Autodesk Inventor part; units mm, degrees
ref_plane "YZ Plane" through (0, 0, 0) normal (1, 0, 0) x (0, 1, 0)
ref_plane "XZ Plane" through (0, 0, 0) normal (0, 1, 0) x (-1, 0, 0)
ref_plane "XY Plane" through (0, 0, 0) normal (0, 0, 1) x (1, 0, 0)
sketch "Sketch1" plane through (0, 0, 0) normal (1, 0, 0) x (0, 1, 0)
  line L0 (-1143.0823, -35.5862) -> (966.1492, 732.1113)
  line L1 (-1143.0823, -35.5862) -> (-1143.0823, -135.5862)
  line L2 (966.1492, 732.1113) -> (966.1492, 632.1113)
  line L3 (-1143.0823, -135.5862) -> (966.1492, 632.1113)
  point P0 (0, 0)
  point P1 (1136.1492, -719.9922)
extrude "Extrusion1" add sketch "Sketch1" along normal blind 1696
sketch "Sketch2" plane through (1696, 0, 0) normal (1, 0, 0) x (0, 0, -1)
  line L0 (-632.1113, 966.1492) -> (-732.1113, 966.1492)
  line L1 (-732.1113, 966.1492) -> (-595.3032, 590.2722)
  line L2 (-595.3032, 590.2722) -> (-585.3032, 590.2722)
  line L3 (-585.3032, 590.2722) -> (-578.4628, 571.4783)
  line L4 (-578.4628, 571.4783) -> (-588.4628, 571.4783)
  line L5 (-588.4628, 571.4783) -> (-451.6548, 195.6013)
  line L6 (-732.1113, 966.1492) -> (35.5862, -1143.0823)
  line L7 (-451.6548, 195.6013) -> (-441.6548, 195.6013)
  line L8 (-441.6548, 195.6013) -> (-434.8144, 176.8074)
  line L9 (-434.8144, 176.8074) -> (-445.1891, 177.8369)
  line L10 (-445.1891, 177.8369) -> (-308.381, -198.0401)
  line L11 (-308.381, -198.0401) -> (-298.381, -198.0401)
  line L12 (-298.381, -198.0401) -> (-291.5406, -216.834)
  line L13 (-291.5406, -216.834) -> (-301.5406, -216.834)
  line L14 (-301.5406, -216.834) -> (-164.7326, -592.711)
  line L15 (-164.7326, -592.711) -> (-154.7326, -592.711)
  line L16 (-154.7326, -592.711) -> (-147.8921, -611.5049)
  line L17 (-147.8921, -611.5049) -> (-157.8921, -611.5049)
  line L18 (-157.8921, -611.5049) -> (-21.0841, -987.3819)
  line L19 (-21.0841, -987.3819) -> (-11.0841, -987.3819)
  line L20 (-11.0841, -987.3819) -> (-4.2437, -1006.1758)
  line L21 (-4.2437, -1006.1758) -> (-14.2437, -1006.1758)
  line L22 (-14.2437, -1006.1758) -> (-595.3032, 590.2722)
  point P0 (0, 0)
  point P1 (-582.1113, 966.1492)
  dimension "d2" = 400
  dimension "d3" = 10
  dimension "d4" = 110
  dimension "d5" = 20
  dimension "d6" = 110
  dimension "d7" = 400
  dimension "d8" = 10
  dimension "d9" = 20
  dimension "d10" = 400
  dimension "d11" = 20
  dimension "d12" = 400
  dimension "d13" = 20
  dimension "d14" = 400
  dimension "d15" = 20
extrude "Extrusion2" cut sketch "Sketch2" against normal through all
fillet "Fillet1" radius 10 10 edges at (848, -1006.1758, 14.2437) (848, -987.3819, 21.0841) (848, -611.5049, 157.8921) (848, -592.711, 164.7326) (848, -216.834, 301.5406) (848, -198.0401, 308.381) (848, 177.8369, 445.1891) (848, 195.6013, 451.6548) (848, 571.4783, 588.4628) (848, 590.2722, 595.3032)
properties part number "side_curve_panel_02" material "Wood (Maple)"
Here's how the part is built. I have some questions about the finished solid (model axes, mm). Give positions to 0.01 mm unless a question says otherwise; leave off trailing zeros. Order: outer loops, then holes, each group sorted by start corner. A loop starts at its lowest first (then second) coordinate and runs counter-clockwise, first axis right, second up. Notation, with made-up numbers: (5.5, 41.25) - (10.5, 41.25) arc R3 cw to (10.5, 45.25) - close; hole circle Ø5 at (79.25, -39). An arc over 180 degrees is marked (long way). Answer as a JSON object with one key per item and string values. Group by question number.
Item 1: If we section it at C-C on y = -661.5: Please give me the cut outline in (x, z).
Item 2: For P1, Ø3, axis at x = 475.5, y = 715, coming from the +Z side; P2, Ø3, axis at x = 1424.5, y = -167.5, coming from the +Z side; P3, Ø3.5, axis at x = 681.5, z = 587.5, coming from the -Y side, each with a flat end and sliding along its axis, tell me the tip position at first contact or that it passes through.
Item 3: Please list where these lines run through material, in increasing order: probe 1 along Z at (x, y) = (1475, 60.5); probe 2 along Z at (x, y) = (597, 743).
Item 4: If we section it at B-B on z = 123: Please give me the cut outline in (x, y).
Result set:
{
 "1": {"outline": "(0, 39.7) - (1696, 39.7) - (1696, 139.7) - (0, 139.7) - close"},
 "2": {"P1": "z = 641.25", "P2": "z = 320.04", "P3": "y = 590.27"},
 "3": {"probe 1": "302.48 to 402.48", "probe 2": "550.89 to 650.89"},
 "4": {"outline": "(0, -707.37) - (1696, -707.37) - (1696, -432.62) - (0, -432.62) - close"}
}
